```python
from build123d import *

# Parameters (mm, degrees)
F3_DEPTH = 8


with BuildPart() as f1:
    # F0 (on Right) → F1 (revolve)
    with BuildSketch(Plane.YZ):
        Polygon((9.525, 18.025), (9.525, 8.025), (1.5, 0), (3.5, 0), (11.525, 8.025), (11.525, 18.025), align=None)
    revolve(axis=Axis((0, 0, 10.187358), (0, 0, 1)))

    # F2 (on face) → F3 (join)
    with BuildSketch(Plane.XY.offset(18.025)):
        with BuildLine():
            ThreePointArc((4.5, -10.610166), (0, -11.525), (-4.5, -10.610166))
            Line((-4.5, -10.610166), (-4.5, -15.025))
            ThreePointArc((-4.5, -15.025), (0, -19.525), (4.5, -15.025))
            Line((4.5, -15.025), (4.5, -10.610166))
        make_face()
        with BuildLine():
            Line((-2.5, -15.025), (-2.5, -12.525))
            Line((-2.5, -12.525), (2.5, -12.525))
            Line((2.5, -12.525), (2.5, -15.025))
            ThreePointArc((2.5, -15.025), (0, -17.525), (-2.5, -15.025))
        make_face(mode=Mode.SUBTRACT)
    extrude(amount=-F3_DEPTH)


solid = f1.part
```
Check sheet for the modelled part. Datum: model origin and axes. Units: mm. A direction names the side the tool comes from. Round coordinates to 2 decimals unless told otherwise and drop trailing zeros. Order: outer loops, then holes, each group sorted by start corner. A loop starts at its lowest first (then second) coordinate and runs counter-clockwise, first axis right, second up.
1) Section check A-A (y = 0). Record the boundary of the cut face in (x, z) (3 decimals), and give its area (3 significant figures).
2) Section check D-D (z = 5). Record the boundary of the cut face in (x, y).
3) Section check B-B (x = 0). Record the boundary of the cut face in (y, z) (3 decimals), and give its area (3 significant figures).
4) Section check C-C (z = 2.25). Record the boundary of the cut face in (x, y).
5) Scan lines: line 1 (Y direction, x = 0, z = 14.5) (3 decimals); line 2 (X direction, y = 0, z = 15) (3 decimals); line 3 (X direction, y = -15, z = 11.25). Record each from-to range of solid material in increasing order.
6) Tool access check on faces 1 (the conical face through (3.9, -0.9, 0.5)), 2 (the cylindrical face through (5.796, -7.559, 12.955)), 3 (the flat face through (2.5, -14, 14)), 4 (the flat face through (4.5, -13, 14)), 5 (the flat face through (-4.5, -13, 14)). Record the directions out of +Z, -Z, +X, -X, +Y, -Y that give a thin tool (end or side, any length) a straight path to the whole face; none if there is none.
7) Mould release check, pull along Y, two halves, no side actions. Record for faces 6 (the cylindrical face through (-0.099, -19.524, 14.081)), 7 (the flat face through (2, -17, 10.025)), 8 (the flat face through (-2.5, -14, 14)), 9 (the cylindrical face through (-3.462, 10.993, 13.095)): +Y half, -Y half, draft (parallel to the pull), parting line (faces both ways), or undercut.
8) Go/stop test with flat-tipped pins: pin 1 Ø4 at (y, z) = (-5.5, 2.5) entering from -X; pin 2 Ø0.8 at (y, z) = (-13, 13.5) entering from +X; pin 3 Ø5 at (x, z) = (6.5, 7.5) entering from +Y. Record where each tip stops, or that it passes through.
Result:
1. outline: (-11.525, 8.025) - (-3.5, 0) - (-1.5, 0) - (-9.525, 8.025) - (-9.525, 18.025) - (-11.525, 18.025) - close; (1.5, 0) - (3.5, 0) - (11.525, 8.025) - (11.525, 18.025) - (9.525, 18.025) - (9.525, 8.025) - close
1. area: 72.1 mm2
2. outline: circle Ø17 at (0, 0); hole circle Ø13 at (0, 0)
3. outline: (-19.525, 10.025) - (-17.525, 10.025) - (-17.525, 18.025) - (-19.525, 18.025) - close; (-12.525, 10.025) - (-11.525, 10.025) - (-11.525, 8.025) - (-3.5, 0) - (-1.5, 0) - (-9.525, 8.025) - (-9.525, 18.025) - (-12.525, 18.025) - close; (1.5, 0) - (3.5, 0) - (11.525, 8.025) - (11.525, 18.025) - (9.525, 18.025) - (9.525, 8.025) - close
3. area: 96.1 mm2
4. outline: circle Ø11.5 at (0, 0); hole circle Ø7.5 at (0, 0)
5. line 1: y = -19.525 to -17.525, -12.525 to -9.525, 9.525 to 11.525
5. line 2: x = -11.525 to -9.525, 9.525 to 11.525
5. line 3: x = -4.5 to -2.5, 2.5 to 4.5
6. face 1: -Z
6. face 2: +Z
6. face 3: +Z, -Z
6. face 4: +Z, -Z, +X, -Y
6. face 5: +Z, -Z, -X, -Y
7. face 6: -Y half
7. face 7: draft
7. face 8: undercut
7. face 9: parting line
8. pin 1: stops at x = -6.29
8. pin 2: stops at x = 4.5
8. pin 3: stops at y = 10.79
